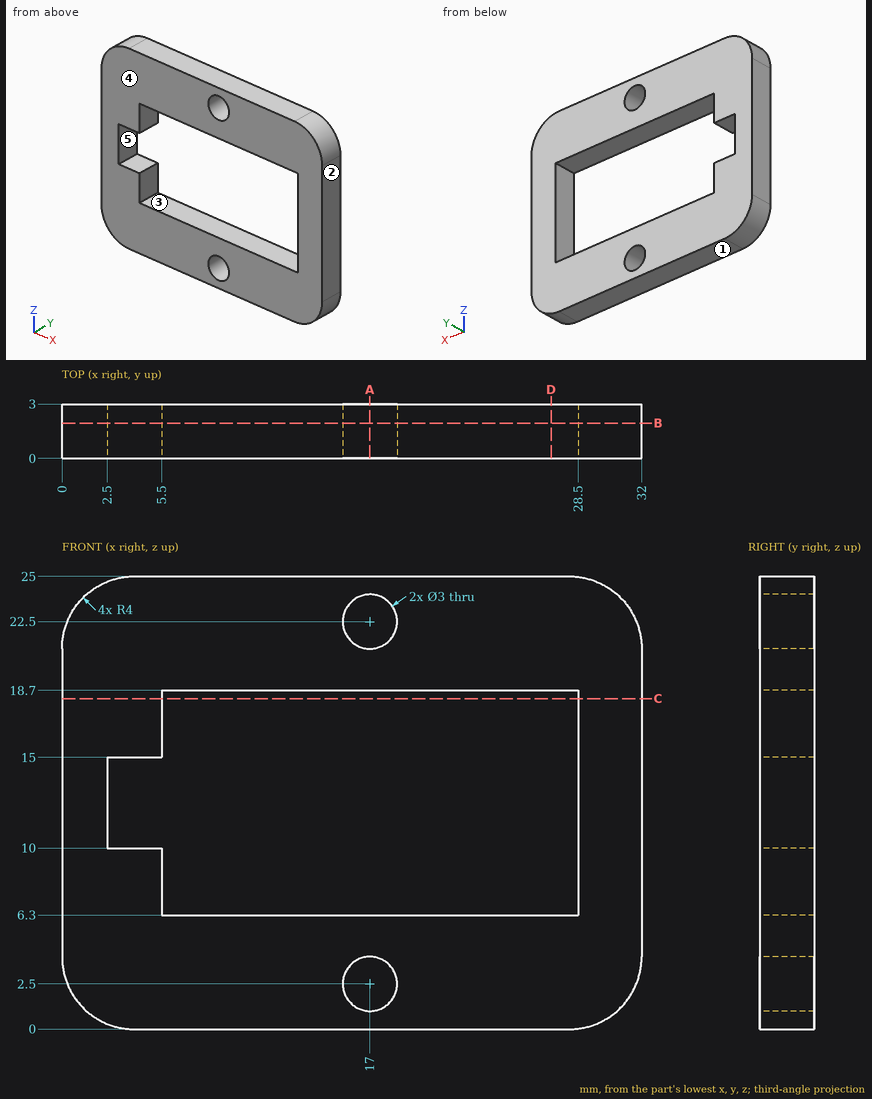
Geometry: see drawing. Coordinates: mm, zero at the bounding-box minimum. A direction names the side the tool comes from. Coordinates: 2 decimals unless noted, no trailing zeros. Order: outer loops, then holes, each group sorted by start corner. A loop starts at its lowest first (then second) coordinate and runs counter-clockwise, first axis right, second up. Notation, with made-up numbers: (-7, -16) - (26, -16) arc R13 cw to (26, 5) - close; hole circle Ø10 at (66.5, 27). An arc over 180 degrees is marked (long way). Write each question's results on one line, items separated by ' | '.
1) Set-up query: the marked faces 4 and 5. Return all of +Z, -Z, +X, -X, +Y, -Y with unobstructed straight access to the full face (end or side cutting, diameter ignored); none if empty.
Results list:
face 4: +Z, -Z, +X, -X, -Y | face 5: +Y, -Y
2) Section D-D, the plane x = 27. Return loops of the section in (y, z).
Results list:
outline: (0, 0) - (3, 0) - (3, 6.3) - (0, 6.3) - close; (0, 18.7) - (3, 18.7) - (3, 25) - (0, 25) - close
3) Section A-A, the plane x = 17. Return loops of the section in (y, z), plus the area to 3 significant figures.
Results list:
outline: (0, 0) - (3, 0) - (3, 1) - (0, 1) - close; (0, 4) - (3, 4) - (3, 6.3) - (0, 6.3) - close; (0, 18.7) - (3, 18.7) - (3, 21) - (0, 21) - close; (0, 24) - (3, 24) - (3, 25) - (0, 25) - close | area: 19.8 mm^2
4) Section B-B, the plane y = 1.95. Return loops of the section in (x, z).
Results list:
outline: (0, 4) arc R4 ccw to (4, 0) - (28, 0) arc R4 ccw to (32, 4) - (32, 21) arc R4 ccw to (28, 25) - (4, 25) arc R4 ccw to (0, 21) - close; hole (2.5, 10) - (5.5, 10) - (5.5, 6.3) - (28.5, 6.3) - (28.5, 18.7) - (5.5, 18.7) - (5.5, 15) - (2.5, 15) - close; hole circle Ø3 at (17, 2.5); hole circle Ø3 at (17, 22.5)
5) Line query: line 1 (Z direction, x = 17, y = 1.2); line 2 (Z direction, x = 22, y = 0.2); line 3 (X direction, y = 2.65, z = 7.75). Output: solid intervals per line, ascending. Write a range as from..to.
Results list:
line 1: 0..1, 4..6.3, 18.7..21, 24..25 | line 2: 0..6.3, 18.7..25 | line 3: 0..5.5, 28.5..32
6) Pull-direction query (X, two-part tool) for the marked faces 1, 2 and 3; classes: pulls with the +X half, pulls with the -X half, needs draft (parallel to the pull), parting line crosses it, or undercut.
Results list:
face 1: needs draft | face 2: pulls with the +X half | face 3: undercut
7) Section C-C, the plane z = 18.25. Return loops of the section in (x, y), plus the area to 3 significant figures.
Results list:
outline: (0, 0) - (5.5, 0) - (5.5, 3) - (0, 3) - close; (28.5, 0) - (32, 0) - (32, 3) - (28.5, 3) - close | area: 27.0 mm^2
